Build history of the part. All positions in model axes, mm. A direction names the side the tool comes from. Give positions to 0.01 mm unless a question says otherwise; leave off trailing zeros. Loops run counter-clockwise (first coordinate to the right, second up) from the corner with the lowest first, then second, coordinate; pieces in that order, holes last.
1) Band-saw the part on C-C on z = -20. List the corners of the cut face in (x, y), then the cut area to 3 significant figures.
2) Flat gauge pins, fed straight in: P1, Ø12, axis at x = 0, y = 0, coming from the +Z side; P2, Ø12, axis at x = 0.5, y = 5, coming from the +Z side; P3, Ø6, axis at x = 0, y = 0, coming from the -Z side (3 decimals). Where does each tip first touch, or does it go through?
3) Band-saw the part on A-A on y = 0. List the corners of the cut face in (x, z), then the cut area to 3 significant figures.
4) Two-plate mould, pull along Y, no slides. Class faces 3 (the flat face through (-1, 50, -25)), 4 (the flat face through (50, -1, -25)), 5 (the cylindrical face through (-19.524, -4.336, -7.754)): +Y half, -Y half, draft (parallel to the pull), parting line (faces both ways), or undercut.
5) Wall check: line 1 (X direction, y = 0, z = -21.5); line 2 (Y direction, x = 0.5, z = -44); line 3 (Y direction, x = -0.5, z = -15). Give the ranges that are in metal, low to high.
6) Band-saw the part on D-D on z = -9.5. List the corners of the cut face in (x, y), then the cut area to 3 significant figures.
7) 3-axis set-ups, long thin cutter, end or side, ignore diameter. For faces 1 (the flat face through (-1, 12, -50)), 2 (the flat face through (9, 5, -15.728)): which of +Z, -Z, +X, -X, +Y, -Y reach the whole face in a straight line?
```python
from build123d import *

# Parameters (mm, degrees)
F0_W     = 100
F0_H     = 100
F1_DEPTH = 50


with BuildPart() as f1:
    # F0 (on Top) → F1 (new body)
    with BuildSketch(Plane.XY):
        Rectangle(F0_W, F0_H)
    extrude(amount=-F1_DEPTH)

    # F2 (on Right) → F3 (revolve, cut)
    with BuildSketch(Plane.YZ):
        Polygon((20, 0), (0, 0), (0, -50), (5, -50), (5, -35.036158), (10, -35.036158), (10, -15.728306), (20, -15.728306), align=None)
    revolve(axis=Axis((0, 0, 12.636881), (0, 0, -1)), mode=Mode.SUBTRACT)


solid = f1.part
```
Findings below:
1. outline: (-50, -50) - (50, -50) - (50, 50) - (-50, 50) - close; hole circle Ø20 at (0, 0)
1. area: 9,690 mm2
2. P1: stops at z = -35.04
2. P2: stops at z = -15.73
2. P3: passes through
3. outline: (-50, -50) - (-5, -50) - (-5, -35.04) - (-10, -35.04) - (-10, -15.73) - (-20, -15.73) - (-20, 0) - (-50, 0) - close; (5, -50) - (50, -50) - (50, 0) - (20, 0) - (20, -15.73) - (10, -15.73) - (10, -35.04) - (5, -35.04) - close
3. area: 3,840 mm2
4. face 3: +Y half
4. face 4: draft
4. face 5: undercut
5. line 1: x = -50 to -10, 10 to 50
5. line 2: y = -50 to -4.97, 4.97 to 50
5. line 3: y = -50 to -19.99, 19.99 to 50
6. outline: (-50, -50) - (50, -50) - (50, 50) - (-50, 50) - close; hole circle Ø40 at (0, 0)
6. area: 8,740 mm2
7. face 1: -Z, +X, -X, +Y, -Y
7. face 2: +Z
